Part model, mm, in its own coordinate system. Face numbers are marked on the shaded views. A direction names the side the tool comes from. Round coordinates to 2 decimals unless told otherwise and drop trailing zeros. Loops run counter-clockwise (first coordinate to the right, second up) from the corner with the lowest first, then second, coordinate; pieces in that order, holes last.
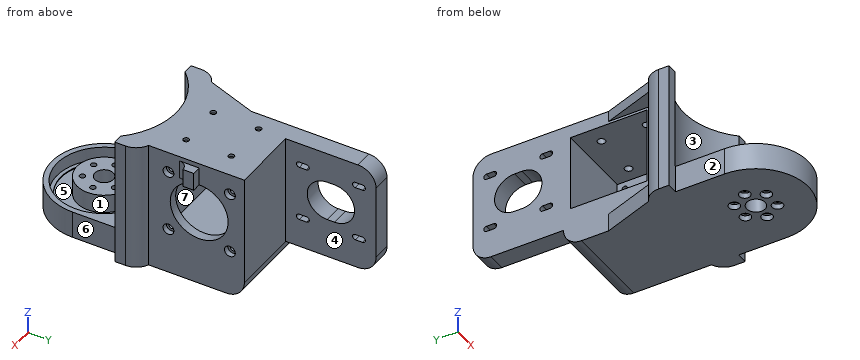
from build123d import *

# Parameters (mm, degrees)
SKETCH_1_R           = 29
EXTRUDE_1_DEPTH      = 15
SKETCH_2_R           = 1.55
SKETCH_2_R_2         = 5.1
CUT_EXTRUDE_1_DEPTH  = 44.669211122
EXTRUDE_2_DEPTH      = 71
SKETCH_12_W          = 70
SKETCH_12_H          = 15
EXTRUDE_3_DEPTH      = 71
FILLET_5_R           = 10
SKETCH_22_W          = 71
SKETCH_22_H          = 103
CUT_EXTRUDE_11_DEPTH = 10
SKETCH_4_R           = 40
CUT_EXTRUDE_2_DEPTH  = 56
SKETCH_5_R           = 16
SKETCH_5_R_2         = 1.55
CUT_EXTRUDE_3_DEPTH  = 171.241005636
SKETCH_6_W           = 42.2
SKETCH_6_H           = 42.2
CUT_EXTRUDE_4_DEPTH  = 43
CUT_EXTRUDE_5_DEPTH  = 171.241005636
SKETCH_8_W           = 10
SKETCH_8_H           = 50
CUT_EXTRUDE_6_DEPTH  = 10
FILLET_1_R           = 10
FILLET_2_R           = 10
FILLET_3_R           = 10
SKETCH_17_R          = 26.1
CUT_EXTRUDE_7_DEPTH  = 7.3
SKETCH_18_R          = 24
CUT_EXTRUDE_8_DEPTH  = 0.5
EXTRUDE_START        = 10.3
SKETCH_19_R          = 15
SKETCH_19_R_2        = 1.55
SKETCH_19_R_3        = 5.1
EXTRUDE_5_DEPTH      = 10.3
SKETCH_20_R          = 3
CUT_EXTRUDE_9_DEPTH  = 3
SKETCH_23_R          = 1.6
CUT_EXTRUDE_12_DEPTH = 163.157207672
SKETCH_26_R          = 2.1
CUT_EXTRUDE_13_DEPTH = 6
SKETCH_27_R          = 3
CUT_EXTRUDE_14_DEPTH = 3
SKETCH_28_W          = 10
SKETCH_28_H          = 6
EXTRUDE_6_DEPTH      = 5
FILLET_6_R           = 5
EXTRUDE_7_DEPTH      = 10
EXTRUDE_8_DEPTH      = 6


# Some blends are built 0.0001 mm under size
with BuildPart() as part:
    # Sketch 1 → Extrude 1 (new body)
    with BuildSketch(Plane.XY):
        Circle(SKETCH_1_R)
    extrude(amount=EXTRUDE_1_DEPTH)

    # Sketch 2 → Cut-Extrude 1 (cut, through all)
    with BuildSketch(Plane.XY.offset(15)):
        with Locations((-5.125, 8.876760389)):
            Circle(SKETCH_2_R)
        with Locations((5.125, 8.876760389)):
            Circle(SKETCH_2_R)
        with Locations((10.25, 0)):
            Circle(SKETCH_2_R)
        with Locations((5.125, -8.876760389)):
            Circle(SKETCH_2_R)
        Circle(SKETCH_2_R_2)
        with Locations((-5.125, -8.876760389)):
            Circle(SKETCH_2_R)
        with Locations((-10.25, 0)):
            Circle(SKETCH_2_R)
    extrude(amount=-CUT_EXTRUDE_1_DEPTH, mode=Mode.SUBTRACT)

    # Sketch 17 → Cut-Extrude 7 (cut)
    with BuildSketch(Plane.XY.offset(15)):
        Circle(SKETCH_17_R)
    extrude(amount=-CUT_EXTRUDE_7_DEPTH, mode=Mode.SUBTRACT)

    # Sketch 18 → Cut-Extrude 8 (cut)
    with BuildSketch(Plane.XY.offset(7.7)):
        Circle(SKETCH_18_R)
    extrude(amount=-CUT_EXTRUDE_8_DEPTH, mode=Mode.SUBTRACT)


with BuildPart() as body_2:
    # Sketch 3 → Extrude 2 (new body)
    with BuildSketch(Plane.XY):
        with BuildLine():
            ThreePointArc((-29, 0), (0, 29), (29, 0))
            Line((29, 0), (29, 95))
            Line((29, 95), (-9, 95))
            Line((-9, 95), (-9, 145))
            Line((-9, 145), (-29, 145))
            Line((-29, 145), (-29, 0))
        make_face()
    extrude(amount=EXTRUDE_2_DEPTH)

    # Sketch 12 → Extrude 3 (add)
    with BuildSketch(Plane.XY.offset(71)):
        with Locations((0, 34.5)):
            Rectangle(SKETCH_12_W, SKETCH_12_H)
    extrude(amount=-EXTRUDE_3_DEPTH)

    # Fillet 5
    # the kernel refuses this fillet: 10 mm, written as the material it takes off along each edge
    with BuildSketch(Plane(origin=(35, 42, 93.912878475), x_dir=(0, -1, 0), z_dir=(0, 0, -1))) as fillet_5_piece_1:
        with BuildLine():
            CenterArc((9.16515139, 10), FILLET_5_R, 203.578178478, 66.421821522)
            Line((0, 6), (-0.183303028, 5.92))
            ThreePointArc((-0.183303028, 5.92), (-0.2, 3), (-0.2, 0))
            Line((-0.2, 0), (0, -0.2))
            Line((0, -0.2), (9.16515139, -0.2))
            Line((9.16515139, -0.2), (9.16515139, 0))
        make_face()
    extrude(amount=116.82575695, mode=Mode.SUBTRACT)
    with BuildSketch(Plane(origin=(-35, 42, 93.912878475), x_dir=(0, -1, 0), z_dir=(0, 0, -1))) as fillet_5_piece_2:
        with BuildLine():
            CenterArc((9.16515139, -10), FILLET_5_R, 90, 66.421821522)
            Line((0, -6), (-0.183303028, -5.92))
            ThreePointArc((-0.183303028, -5.92), (-0.2, -3), (-0.2, 0))
            Line((-0.2, 0), (0, 0.2))
            Line((0, 0.2), (9.16515139, 0.2))
            Line((9.16515139, 0.2), (9.16515139, 0))
        make_face()
    extrude(amount=116.82575695, mode=Mode.SUBTRACT)

    # Sketch 22 → Cut-Extrude 11 (cut)
    with BuildSketch(Plane.ZY.offset(29)):
        with Locations((35.5, 93.5)):
            Rectangle(SKETCH_22_W, SKETCH_22_H)
    extrude(amount=-CUT_EXTRUDE_11_DEPTH, mode=Mode.SUBTRACT)

    # Sketch 4 → Cut-Extrude 2 (cut)
    with BuildSketch(Plane.XY.offset(71)):
        Circle(SKETCH_4_R)
    extrude(amount=-CUT_EXTRUDE_2_DEPTH, mode=Mode.SUBTRACT)

    # Sketch 5 → Cut-Extrude 3 (cut, through all)
    with BuildSketch(Plane.ZY.offset(19)):
        with Locations(Location((42.5, 70, 0), (0, 0, 270))):
            Circle(SKETCH_5_R)
        with Locations(Location((25.529437252, 86.970562748, 0), (0, 0, 270))):
            Circle(SKETCH_5_R_2)
        with Locations(Location((59.470562748, 86.970562748, 0), (0, 0, 270))):
            Circle(SKETCH_5_R_2)
        with Locations(Location((59.470562748, 53.029437252, 0), (0, 0, 270))):
            Circle(SKETCH_5_R_2)
        with Locations(Location((25.529437252, 53.029437252, 0), (0, 0, 270))):
            Circle(SKETCH_5_R_2)
    extrude(amount=-CUT_EXTRUDE_3_DEPTH, mode=Mode.SUBTRACT)

    # Sketch 6 → Cut-Extrude 4 (cut)
    with BuildSketch(Plane.ZY.offset(19)):
        with Locations((42.5, 70)):
            Rectangle(SKETCH_6_W, SKETCH_6_H)
    extrude(amount=-CUT_EXTRUDE_4_DEPTH, mode=Mode.SUBTRACT)

    # Sketch 7 → Cut-Extrude 5 (cut, through all)
    with BuildSketch(Plane.ZY.offset(19)):
        with BuildLine():
            Line((56.95, 137.497499937), (56.95, 133.497499937))
            ThreePointArc((56.95, 133.497499937), (58.5, 131.947499937), (60.05, 133.497499937))
            Line((60.05, 133.497499937), (60.05, 137.497499937))
            ThreePointArc((60.05, 137.497499937), (58.5, 139.047499937), (56.95, 137.497499937))
        make_face()
        with BuildLine():
            Line((54.1, 121.997499937), (54.1, 117.997499937))
            ThreePointArc((54.1, 117.997499937), (43, 106.897499937), (31.9, 117.997499937))
            Line((31.9, 117.997499937), (31.9, 121.997499937))
            ThreePointArc((31.9, 121.997499937), (43, 133.097499937), (54.1, 121.997499937))
        make_face()
        with BuildLine():
            Line((29.05, 137.497499937), (29.05, 133.497499937))
            ThreePointArc((29.05, 133.497499937), (27.5, 131.947499937), (25.95, 133.497499937))
            Line((25.95, 133.497499937), (25.95, 137.497499937))
            ThreePointArc((25.95, 137.497499937), (27.5, 139.047499937), (29.05, 137.497499937))
        make_face()
        with BuildLine():
            Line((56.95, 106.497499937), (56.95, 102.497499937))
            ThreePointArc((56.95, 102.497499937), (58.5, 100.947499937), (60.05, 102.497499937))
            Line((60.05, 102.497499937), (60.05, 106.497499937))
            ThreePointArc((60.05, 106.497499937), (58.5, 108.047499937), (56.95, 106.497499937))
        make_face()
        with BuildLine():
            Line((25.95, 106.497499937), (25.95, 102.497499937))
            ThreePointArc((25.95, 102.497499937), (27.5, 100.947499937), (29.05, 102.497499937))
            Line((29.05, 102.497499937), (29.05, 106.497499937))
            ThreePointArc((29.05, 106.497499937), (27.5, 108.047499937), (25.95, 106.497499937))
        make_face()
    extrude(amount=-CUT_EXTRUDE_5_DEPTH, mode=Mode.SUBTRACT)

    # Sketch 8 → Cut-Extrude 6 (cut)
    with BuildSketch(Plane(origin=(0, 0, 0), x_dir=(-1, 0, 0), z_dir=(0, 0, -1))):
        with Locations((14, 120)):
            Rectangle(SKETCH_8_W, SKETCH_8_H)
    extrude(amount=-CUT_EXTRUDE_6_DEPTH, mode=Mode.SUBTRACT)

    # Fillet 1
    fillet_1_edges = [body_2.edges().sort_by_distance(p)[0] for p in [
        (5, 95, 0),
    ]]
    fillet(fillet_1_edges, radius=FILLET_1_R)

    # Fillet 2
    fillet_2_edges = [body_2.edges().sort_by_distance(p)[0] for p in [
        (-14, 145, 10),
    ]]
    fillet(fillet_2_edges, radius=FILLET_2_R)

    # Fillet 3
    fillet_3_edges = [body_2.edges().sort_by_distance(p)[0] for p in [
        (-14, 145, 71),
    ]]
    fillet(fillet_3_edges, radius=FILLET_3_R)


    add(part.part)  # Extrude 5 merges part
    # Sketch 19 → Extrude 5 (add)
    with BuildSketch(Plane.XY.offset(7.2).offset(EXTRUDE_START)):
        with Locations(Location((0, 0, 0), (0, 0, 180))):
            Circle(SKETCH_19_R)
        with Locations((-5.125, -8.876760389)):
            Circle(SKETCH_19_R_2, mode=Mode.SUBTRACT)
        with Locations((5.125, -8.876760389)):
            Circle(SKETCH_19_R_2, mode=Mode.SUBTRACT)
        with Locations((10.25, 0)):
            Circle(SKETCH_19_R_2, mode=Mode.SUBTRACT)
        Circle(SKETCH_19_R_3, mode=Mode.SUBTRACT)
        with Locations((5.125, 8.876760389)):
            Circle(SKETCH_19_R_2, mode=Mode.SUBTRACT)
        with Locations((-5.125, 8.876760389)):
            Circle(SKETCH_19_R_2, mode=Mode.SUBTRACT)
        with Locations((-10.25, 0)):
            Circle(SKETCH_19_R_2, mode=Mode.SUBTRACT)
    extrude(amount=-EXTRUDE_5_DEPTH)

    # Sketch 20 → Cut-Extrude 9 (cut)
    with BuildSketch(Plane(origin=(0, 0, 0), x_dir=(-1, 0, 0), z_dir=(0, 0, -1))):
        with Locations((-5.125, 8.876760389)):
            Circle(SKETCH_20_R)
        with Locations((5.125, 8.876760389)):
            Circle(SKETCH_20_R)
        with Locations((-10.25, 0)):
            Circle(SKETCH_20_R)
        with Locations((-5.125, -8.876760389)):
            Circle(SKETCH_20_R)
        with Locations((5.125, -8.876760389)):
            Circle(SKETCH_20_R)
        with Locations((10.25, 0)):
            Circle(SKETCH_20_R)
    extrude(amount=-CUT_EXTRUDE_9_DEPTH, mode=Mode.SUBTRACT)

    # Sketch 23 → Cut-Extrude 12 (cut, through all)
    with BuildSketch(Plane(origin=(0, 0, 63.6), x_dir=(-1, 0, 0), z_dir=(0, 0, -1))):
        with Locations((-16, 80)):
            Circle(SKETCH_23_R)
        with Locations((9, 80)):
            Circle(SKETCH_23_R)
        with Locations((9, 55)):
            Circle(SKETCH_23_R)
        with Locations((-16, 55)):
            Circle(SKETCH_23_R)
    extrude(amount=-CUT_EXTRUDE_12_DEPTH, mode=Mode.SUBTRACT)

    # Sketch 26 → Cut-Extrude 13 (cut)
    with BuildSketch(Plane(origin=(0, 0, 63.6), x_dir=(-1, 0, 0), z_dir=(0, 0, -1))):
        with Locations((-16, 80)):
            Circle(SKETCH_26_R)
        with Locations((9, 80)):
            Circle(SKETCH_26_R)
        with Locations((-16, 55)):
            Circle(SKETCH_26_R)
        with Locations((9, 55)):
            Circle(SKETCH_26_R)
    extrude(amount=-CUT_EXTRUDE_13_DEPTH, mode=Mode.SUBTRACT)

    # Sketch 27 → Cut-Extrude 14 (cut)
    with BuildSketch(Plane(origin=(29, 0, 0), x_dir=(0, 0, -1), z_dir=(1, 0, 0))):
        with Locations((-59.470562748, 86.970562748)):
            Circle(SKETCH_27_R)
        with Locations((-25.529437252, 86.970562748)):
            Circle(SKETCH_27_R)
        with Locations((-59.470562748, 53.029437252)):
            Circle(SKETCH_27_R)
        with Locations((-25.529437252, 53.029437252)):
            Circle(SKETCH_27_R)
    extrude(amount=-CUT_EXTRUDE_14_DEPTH, mode=Mode.SUBTRACT)

    # Sketch 28 → Extrude 6 (add)
    with BuildSketch(Plane(origin=(29, 0, 0), x_dir=(0, 0, -1), z_dir=(1, 0, 0))):
        with Locations((-63.5, 67)):
            Rectangle(SKETCH_28_W, SKETCH_28_H)
    extrude(amount=EXTRUDE_6_DEPTH)

    # Fillet 6
    fillet_6_edges = [body_2.edges().sort_by_distance(p)[0] for p in [
        (29, 64, 63.5),
    ]]
    fillet(fillet_6_edges, radius=FILLET_6_R - 0.0001)  # a hair under: the kernel refuses the full size

    # Sketch 29 → Extrude 7 (add)
    with BuildSketch(Plane(origin=(0, 0, 0), x_dir=(-1, 0, 0), z_dir=(0, 0, -1))):
        Polygon((19, 70), (29, 42), (19, 42), align=None)
    extrude(amount=-EXTRUDE_7_DEPTH)

    # Sketch 30 → Extrude 8 (add)
    with BuildSketch(Plane.XY.offset(71)):
        Polygon((-29, 42), (-19, 70), (-19, 42), align=None)
    extrude(amount=-EXTRUDE_8_DEPTH)


solid = body_2.part
1) Slice it at C-C, the plane z = 38.5. Give the cut face in (x, y).
Values:
outline: (-35, 27) - (-29.51, 27) arc R40 cw to (29.51, 27) - (35, 27) - (35, 32.83) arc R10 ccw to (29, 42) - (29, 54.51) - (24, 54.51) - (24, 48.9) - (-19, 48.9) - (-19, 42) - (-29, 42) arc R10 ccw to (-35, 32.83) - close; (-19, 91.1) - (24, 91.1) - (24, 85.49) - (29, 85.49) - (29, 95) - (-9, 95) - (-9, 107.85) - (-19, 107.85) - close; (-19, 132.14) - (-9, 132.14) - (-9, 145) - (-19, 145) - close
2) Mould opens along X. For the marked faces 1, 2, 3 and 4 say: released by +X, released by -X, zero draft, split by the parting line, or undercut.
Values:
face 1: undercut
face 2: released by -X
face 3: undercut
face 4: released by +X
3) Slice it at B-B, the plane y = 67. Give the cut face in (x, z), then the cut area to 3 significant figures.
Values:
outline: (-20.07, 0) - (29, 0) - (29, 26.78) - (24, 26.78) - (24, 21.4) - (-19, 21.4) - (-19, 10) - (-20.07, 10) - close; (-20.07, 65) - (-19, 65) - (-19, 63.6) - (24, 63.6) - (24, 58.22) - (29, 58.22) - (29, 58.5) - (34, 58.5) - (34, 68.5) - (29, 68.5) - (29, 71) - (-20.07, 71) - close
area: 1,500 mm2
4) Slice it at A-A, the plane z = 50. Give the cut face in (x, y).
Values:
outline: (-35, 27) - (-29.51, 27) arc R40 cw to (29.51, 27) - (35, 27) - (35, 32.83) arc R10 ccw to (29, 42) - (29, 55.87) - (24, 55.87) - (24, 48.9) - (-19, 48.9) - (-19, 42) - (-29, 42) arc R10 ccw to (-35, 32.83) - close; (-19, 91.1) - (24, 91.1) - (24, 84.13) - (29, 84.13) - (29, 95) - (-9, 95) - (-9, 109.38) - (-19, 109.38) - close; (-19, 130.61) - (-9, 130.61) - (-9, 145) - (-19, 145) - close
5) Drop flat-ended pins along their axis: pin 1 Ø4 at (y, z) = (86.97, 59.47) entering from +X; pin 2 Ø2.5 at (x, y) = (32, 62.5) entering from -Z; pin 3 Ø12 at (x, z) = (-20, 9) entering from +Y. Give the stop position or say it passes through.
Values:
pin 1: stops at x = 26
pin 2: stops at z = 58.5
pin 3: stops at y = 143.61
6) Tool access for the marked faces 5, 6 and 7: list every direction of +Z, -Z, +X, -X, +Y, -Y with a clear straight run to the whole face (end or side of a thin tool).
Values:
face 5: +Z
face 6: +Z, -Z, +X, -Y
face 7: -X
7) Wall check: line 1 along Y through (x, z) = (-0.5, 11.5); line 2 along Y through (x, z) = (16, 66.45); line 3 along Y through (x, z) = (-13.5, 39). Give the ranges that are in metal, low to high.
Values:
line 1: y = -29 to -26.1, -14.99 to -5.08, 5.08 to 14.99, 26.1 to 95
line 2: y = 36.66 to 52.9, 57.1 to 77.9, 82.1 to 95
line 3: y = 37.65 to 48.9, 91.1 to 107.64, 132.35 to 145
